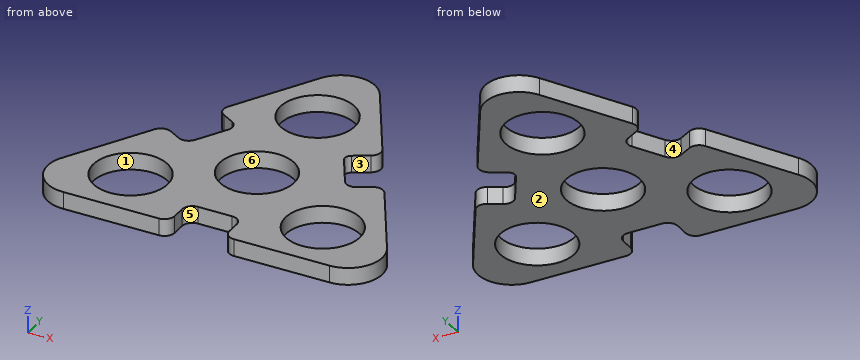
from build123d import *

# Parameters (mm, degrees)
F0_R     = 10.85
F1_DEPTH = 5
F2_R     = 10


with BuildPart() as f1:
    # F0 (on Top) → F1 (new body)
    with BuildSketch(Plane.XY):
        with BuildLine():
            Line((11, -32.5), (42.435245, -32.5))
            Line((42.435245, -32.5), (56.291651, -32.5))
            Line((56.291651, -32.5), (51.528512, -24.25))
            Line((51.528512, -24.25), (33.645826, 6.723721))
            ThreePointArc((33.645826, 6.723721), (31.824207, 8.121498), (29.547749, 7.821797))
            Line((29.547749, 7.821797), (26.083648, 5.821797))
            ThreePointArc((26.083648, 5.821797), (23.807191, 5.522096), (21.985572, 6.919873))
            Line((21.985572, 6.919873), (16.485572, 16.446152))
            ThreePointArc((16.485572, 16.446152), (16.285771, 17.963791), (17.217622, 19.178203))
            Line((17.217622, 19.178203), (21.547749, 21.678203))
            ThreePointArc((21.547749, 21.678203), (22.945527, 23.499822), (22.645826, 25.776279))
            Line((22.645826, 25.776279), (4.76314, 56.75))
            Line((4.76314, 56.75), (0, 65))
            Line((0, 65), (-4.76314, 56.75))
            Line((-4.76314, 56.75), (-22.645826, 25.776279))
            ThreePointArc((-22.645826, 25.776279), (-22.945527, 23.499822), (-21.547749, 21.678203))
            Line((-21.547749, 21.678203), (-18.083648, 19.678203))
            ThreePointArc((-18.083648, 19.678203), (-16.68587, 17.856584), (-16.985572, 15.580127))
            Line((-16.985572, 15.580127), (-21.985572, 6.919873))
            ThreePointArc((-21.985572, 6.919873), (-23.807191, 5.522096), (-26.083648, 5.821797))
            Line((-26.083648, 5.821797), (-29.547749, 7.821797))
            ThreePointArc((-29.547749, 7.821797), (-31.824207, 8.121498), (-33.645826, 6.723721))
            Line((-33.645826, 6.723721), (-51.528512, -24.25))
            Line((-51.528512, -24.25), (-56.291651, -32.5))
            Line((-56.291651, -32.5), (-21.644953, -32.5))
            Line((-21.644953, -32.5), (-11, -32.5))
            ThreePointArc((-11, -32.5), (-8.87868, -31.62132), (-8, -29.5))
            Line((-8, -29.5), (-8, -25.5))
            ThreePointArc((-8, -25.5), (-7.12132, -23.37868), (-5, -22.5))
            Line((-5, -22.5), (5, -22.5))
            ThreePointArc((5, -22.5), (7.12132, -23.37868), (8, -25.5))
            Line((8, -25.5), (8, -29.5))
            ThreePointArc((8, -29.5), (8.87868, -31.62132), (11, -32.5))
        make_face()
        with Locations((-28.145826, -16.25)):
            Circle(F0_R, mode=Mode.SUBTRACT)
        with Locations((28.145826, -16.25)):
            Circle(F0_R, mode=Mode.SUBTRACT)
        Circle(F0_R, mode=Mode.SUBTRACT)
        with Locations((0, 32.5)):
            Circle(F0_R, mode=Mode.SUBTRACT)
    extrude(amount=F1_DEPTH)

    # F2
    f2_edges = [f1.edges().sort_by_distance(p)[0] for p in [
        (56.291651, -32.5, 2.5),
        (0, 65, 2.5),
        (-56.291651, -32.5, 2.5),
    ]]
    fillet(f2_edges, radius=F2_R)


solid = f1.part
Can you work these out from the model? Positions are in its coordinate system, mm. Face numbers are marked on the shaded views. A direction names the side the tool comes from. Round coordinates to 2 decimals unless told otherwise and drop trailing zeros. Loops run counter-clockwise (first coordinate to the right, second up) from the corner with the lowest first, then second, coordinate; pieces in that order, holes last. Notation, with made-up numbers: (56, 59) - (69, 59) arc R10 cw to (69, 66) - close; hole circle Ø4 at (-18.75, -39). An arc over 180 degrees is marked (long way). Answer in a Markdown table with one row per item. Add a question column.
Q1. We'd pull the mould along X, two halves only. Please class the marked faces 1, 2, 3 and 4: pulls with the +X half, pulls with the -X half, needs draft (parallel to the pull), parting line crosses it, or undercut.
Q2. I want a section at C-C on z = 3.3. Count the separate pieces of the cut face and the enclosed holes in it, and give its area (3 significant figures).
Q3. Which directions (+Z, -Z, +X, -X, +Y, -Y) give clear straight access to the entire face, cutting with the end or side of a thin tool? Please do the marked faces 5 and 6.
Q4. For pin 1 Ø12 at (x, y) = (4, -3) entering from +Z; pin 2 Ø1.5 at (x, z) = (21.5, 2.5) entering from +Y; pin 3 Ø2 at (y, z) = (-27.5, 1.5) entering from +X; pin 4 Ø2 at (y, z) = (38.5, 1.5) entering from -X, each with a flat end and sliding along its axis, tell me the tip position at first contact or that it passes through.
Q5. I want a section at A-A on y = 0. List the corners of the cut face in (x, z) for me, and give its area (3 significant figures).
Q6. I want a section at B-B on x = 20. List the corners of the cut face in (y, z) for me.
Q7. I need wall thicknesses on L1, parallel to Y at x = 0, z = 1.05; L2, parallel to Y at x = -28, z = 3.1; L3, parallel to Y at x = -10, z = 1.7. Which ranges of each line are inside material? Lowest first, please.
A:
| question | item | result |
|---|---|---|
| 1 | face 1 | undercut |
| 1 | face 2 | needs draft |
| 1 | face 3 | pulls with the +X half |
| 1 | face 4 | undercut |
| 2 | separate pieces | 1 |
| 2 | enclosed holes | 4 |
| 2 | area | 3,320 mm^2 |
| 3 | face 5 | +Z, -Z, -Y |
| 3 | face 6 | +Z, -Z |
| 4 | pin 1 | z = 5 |
| 4 | pin 2 | y = 29.06 |
| 4 | pin 3 | x = 48.14 |
| 4 | pin 4 | x = -15.88 |
| 5 | outline | (-37.53, 0) - (-10.85, 0) - (-10.85, 5) - (-37.53, 5) - close; (10.85, 0) - (37.53, 0) - (37.53, 5) - (10.85, 5) - close |
| 5 | area | 267 mm^2 |
| 6 | outline | (-32.5, 0) - (-23.42, 0) - (-23.42, 5) - (-32.5, 5) - close; (-9.08, 0) - (10.36, 0) - (10.36, 5) - (-9.08, 5) - close; (20.78, 0) - (30.36, 0) - (30.36, 5) - (20.78, 5) - close |
| 7 | L1 | -22.5 to -10.85, 10.85 to 21.65, 43.35 to 55 |
| 7 | L2 | -32.5 to -27.1, -5.4 to 6.93 |
| 7 | L3 | -32.33 to -4.21, 4.21 to 28.29, 36.71 to 47.68 |
